Check sheet for the modelled part. Datum: model origin and axes. Units: mm. A direction names the side the tool comes from. Give positions to 0.01 mm unless a question says otherwise; leave off trailing zeros. Loops run counter-clockwise (first coordinate to the right, second up) from the corner with the lowest first, then second, coordinate; pieces in that order, holes last. Notation, with made-up numbers: (-1.5, 25) -> (52.5, 25) arc R15 ccw to (52.5, 44) -> close; hole circle Ø8 at (61, 44.25). An arc over 180 degrees is marked (long way). Answer as CSV lines item,"result". Start each with the question number.
(1) Section check D-D on y = 3. Enter the section's corners in (x, z), plus the area to 3 significant figures.
(2) Release check for a two-part mould opening along Z. For faces 1 (the face through (56.4, 17, 0)), 2 (the face through (1, 17, 26.4)), 3 (the face through (56.56, 0.74, -27.7)) record: pulls with the +Z half, pulls with the -Z half, needs draft (parallel to the pull), parting line crosses it, or undercut.
(3) Section check C-C on x = 52. Enter the section's corners in (y, z), plus the area to 3 significant figures.
(4) Access from +Z, -Z, +X, -X, +Y, -Y to the whole of each face (thin tool, end or side, straight path). Record for faces 4 (the face through (-1, 17, -26.4)), 5 (the face through (1, 32, 0)), 6 (the face through (-56.4, 17, 0)).
(5) Section check A-A on x = -58.5. Enter the section's corners in (y, z).
(6) Material ranges on line 1 (X direction, y = 1.1, z = -28.5); line 2 (X direction, y = 10, z = 3); line 3 (Z direction, x = 20.5, y = 10), recorded low to high. Write a range as from..to.
(7) Section check B-B on z = -28.5. Enter the section's corners in (x, y).
(8) Gauge pin test, flat ends, axial feed: pin 1 Ø15 at (y, z) = (21, -6) entering from +X; pin 2 Ø0.6 at (x, y) = (-55, 16) entering from +Z; pin 3 Ø6 at (x, y) = (-40, 6.5) entering from +Z. Record the tip position at first contact, or that the pin passes through.
from build123d import *

# Parameters (mm, degrees)
SKETCH_1_W        = 125
SKETCH_1_H        = 65.5
EXTRUDE_1_DEPTH   = 1.5
HOLE_WIZARD_M41_D = 4.2
EXTRUDE_2_DEPTH   = 30.5


with BuildPart() as part:
    # Эскиз1 → Бобышка-Вытянуть1 (new body)
    with BuildSketch(Plane(origin=(0, 0, 0), x_dir=(1, 0, 0), z_dir=(0, 1, 0))):
        Rectangle(SKETCH_1_W, SKETCH_1_H)
    extrude(amount=EXTRUDE_1_DEPTH)

    # Сверло под метчик  спиральное M41 (through all)
    with Locations(Plane(origin=(0, 1.5, 0), x_dir=(1, 0, 0), z_dir=(0, 1, 0))):
        with Locations((-58.5, -28.5), (-58.5, 28.5), (58.5, 28.5), (58.5, -28.5)):
            Hole(HOLE_WIZARD_M41_D / 2)

    # Эскиз6 → Бобышка-Вытянуть2 (add)
    with BuildSketch(Plane(origin=(0, 1.5, 0), x_dir=(1, 0, 0), z_dir=(0, 1, 0))):
        Polygon((56.4, -24.4), (54.4, -24.4), (54.4, -26.4), (-54.4, -26.4), (-54.4, -24.4), (-56.4, -24.4), (-56.4, 24.4), (-54.4, 24.4), (-54.4, 26.4), (54.4, 26.4), (54.4, 24.4), (56.4, 24.4), align=None)
    extrude(amount=EXTRUDE_2_DEPTH)


solid = part.part
Working result:
1,outline,"(-56.4, -24.4) -> (-54.4, -24.4) -> (-54.4, -26.4) -> (54.4, -26.4) -> (54.4, -24.4) -> (56.4, -24.4) -> (56.4, 24.4) -> (54.4, 24.4) -> (54.4, 26.4) -> (-54.4, 26.4) -> (-54.4, 24.4) -> (-56.4, 24.4) -> close"
1,area,"5,940 mm^2"
2,face 1,"needs draft"
2,face 2,"pulls with the +Z half"
2,face 3,"undercut"
3,outline,"(0, -32.75) -> (1.5, -32.75) -> (1.5, -26.4) -> (32, -26.4) -> (32, 26.4) -> (1.5, 26.4) -> (1.5, 32.75) -> (0, 32.75) -> close"
3,area,"1,710 mm^2"
4,face 4,"-Z, +X, -X, +Y"
4,face 5,"+Z, -Z, +X, -X, +Y"
4,face 6,"+Z, -Z, -X, +Y"
5,outline,"(0, -32.75) -> (1.5, -32.75) -> (1.5, -30.6) -> (0, -30.6) -> close; (0, -26.4) -> (1.5, -26.4) -> (1.5, 26.4) -> (0, 26.4) -> close; (0, 30.6) -> (1.5, 30.6) -> (1.5, 32.75) -> (0, 32.75) -> close"
6,line 1,"x = -62.5..-60.6, -56.4..56.4, 60.6..62.5"
6,line 2,"x = -56.4..56.4"
6,line 3,"z = -26.4..26.4"
7,outline,"(-62.5, 0) -> (-60.6, 0) -> (-60.6, 1.5) -> (-62.5, 1.5) -> close; (-56.4, 0) -> (56.4, 0) -> (56.4, 1.5) -> (-56.4, 1.5) -> close; (60.6, 0) -> (62.5, 0) -> (62.5, 1.5) -> (60.6, 1.5) -> close"
8,pin 1,"stops at x = 56.4"
8,pin 2,"stops at z = 24.4"
8,pin 3,"stops at z = 26.4"
